Design review of the part shown in the three views and the two pictorial views. Dimensions are in mm from the part's minimum x, y and z. Round coordinates to 2 decimals unless told otherwise and drop trailing zeros. Order: outer loops, then holes, each group sorted by start corner. A loop starts at its lowest first (then second) coordinate and runs counter-clockwise, first axis right, second up.
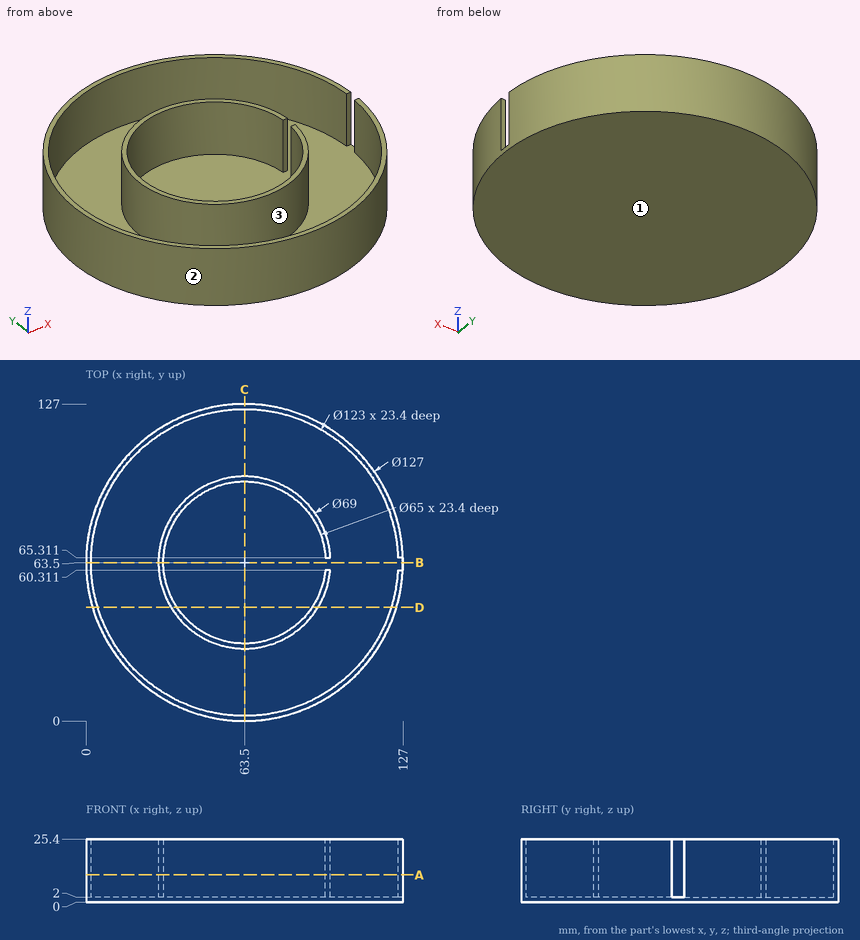
(1) Insertion check: pin 1 (2 mm diameter, centred on y = 73, z = 22.5, fed in from -X); pin 2 (6 mm diameter, centred on x = 104.5, y = 43.5, fed in from +Z); pin 3 (2 mm diameter, centred on x = 66, z = 15, fed in from -Y). Each pin has a flat end and moves straight along its axis. Give the tip position at first contact, or say it passes through.
Data:
pin 1: stops at x = 0.57
pin 2: stops at z = 2
pin 3: stops at y = 0.02
(2) Consider section C-C (x = 63.5). Write out the cut boundary in (y, z).
Data:
outline: (0, 0) - (127, 0) - (127, 25.4) - (125, 25.4) - (125, 2) - (98, 2) - (98, 25.4) - (96, 25.4) - (96, 2) - (31, 2) - (31, 25.4) - (29, 25.4) - (29, 2) - (2, 2) - (2, 25.4) - (0, 25.4) - close
(3) Consider section B-B (y = 63.5). Write out the cut boundary in (x, z), and give its area (3 significant figures).
Data:
outline: (0, 0) - (127, 0) - (127, 2) - (31, 2) - (31, 25.4) - (29, 25.4) - (29, 2) - (2, 2) - (2, 25.4) - (0, 25.4) - close
area: 348 mm2
(4) To check wall thickness, follow probe 1 along Y at (x, z) = (63.5, 10.75); probe 2 along X at (y, z) = (63.5, 13.5); probe 3 along Y at (x, z) = (61.5, 5.25). State the ranges of each line that lie inside material, in increasing order.
Data:
probe 1: y = 0 to 2, 29 to 31, 96 to 98, 125 to 127
probe 2: x = 0 to 2, 29 to 31
probe 3: y = 0.03 to 2.03, 29.06 to 31.06, 95.94 to 97.94, 124.97 to 126.97
(5) Draft analysis for pull direction Y (two halves, no side actions). For the marked faces 1, 2 and 3, state which applies: pulls with the +Y half, pulls with the -Y half, needs draft (parallel to the pull), parting line crosses it, or undercut.
Data:
face 1: needs draft
face 2: parting line crosses it
face 3: undercut
(6) Consider section A-A (z = 11). Write out the cut boundary in (x, y).
Data:
outline: (95.84, 60.31) arc R32.5 cw (long way) to (95.95, 65.31) - (97.95, 65.31) arc R34.5 ccw (long way) to (97.85, 60.31) - close; (124.92, 60.31) arc R61.5 cw (long way) to (124.97, 65.31) - (126.97, 65.31) arc R63.5 ccw (long way) to (126.92, 60.31) - close
(7) Consider section D-D (y = 45.5). Write out the cut boundary in (x, z).
Data:
outline: (2.6, 0) - (124.4, 0) - (124.4, 25.4) - (122.31, 25.4) - (122.31, 2) - (92.93, 2) - (92.93, 25.4) - (90.56, 25.4) - (90.56, 2) - (36.44, 2) - (36.44, 25.4) - (34.07, 25.4) - (34.07, 2) - (4.69, 2) - (4.69, 25.4) - (2.6, 25.4) - close
